Geometry: final body of the model. Coordinates: model frame, mm. Face numbers are marked on the shaded views. A direction names the side the tool comes from. Coordinates: 2 decimals unless noted, no trailing zeros. Loops run counter-clockwise (first coordinate to the right, second up) from the corner with the lowest first, then second, coordinate; pieces in that order, holes last. Notation, with made-up numbers: (58, 47) -> (88, 47) arc R27 cw to (88, 79) -> close; hole circle Ø2 at (72, -26). An arc over 180 degrees is marked (long way). One line per item, written item: value. Start each with the question number.
Item 1: Set-up query: the marked faces 1, 2, 3, 4 and 5. Return all of +Z, -Z, +X, -X, +Y, -Y with unobstructed straight access to the full face (end or side cutting, diameter ignored); none if empty.
Item 2: Section query C-C on x = 2.3. Return loops of the section in (y, z).
Item 3: Section query A-A on x = 3. Return loops of the section in (y, z), then the cut area to 3 significant figures.
Item 4: Section query D-D on x = -0.9. Return loops of the section in (y, z), then the cut area to 3 significant figures.
Item 5: Section query B-B on z = 1.55. Return loops of the section in (x, y).
Item 6: Ray query, probe 1 along Y at (x, z) = (2.1, 2.7); probe 2 along X at (y, z) = (-1.8, 0.2); probe 3 along Z at (x, y) = (1.35, 2.15). Return the intervals inside material, ascending. Write a range as from..to.
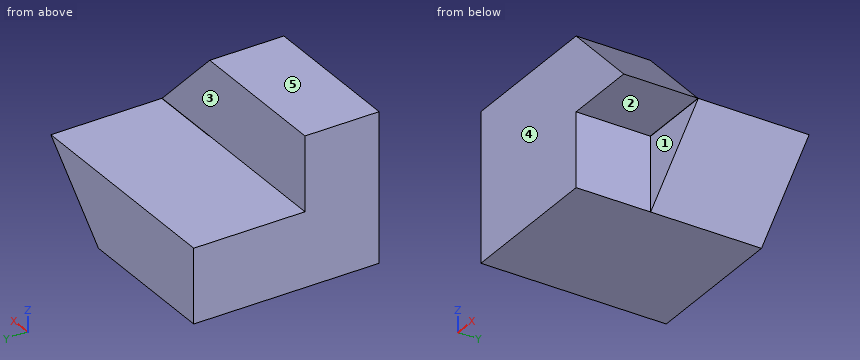
from build123d import *

# Parameters (mm, degrees)
SKETCH1_W           = 4
SKETCH1_H           = 5
BOSS_EXTRUDE1_DEPTH = 2
SKETCH2_W           = 4
SKETCH2_H           = 2
BOSS_EXTRUDE2_DEPTH = 2
BOSS_EXTRUDE3_DEPTH = 2
BOSS_EXTRUDE5_DEPTH = 2.99


with BuildPart() as part:
    # Sketch1 → Boss-Extrude1 (new body)
    with BuildSketch(Plane.XY):
        Rectangle(SKETCH1_W, SKETCH1_H)
    extrude(amount=BOSS_EXTRUDE1_DEPTH)

    # Sketch2 → Boss-Extrude2 (add)
    with BuildSketch(Plane.XY.offset(2)):
        with Locations((0, -1.5)):
            Rectangle(SKETCH2_W, SKETCH2_H)
    extrude(amount=BOSS_EXTRUDE2_DEPTH)

    # Sketch3 → Boss-Extrude3 (add)
    with BuildSketch(Plane(origin=(0, -0.5, 0), x_dir=(1, 0, 0), z_dir=(0, 1, 0))):
        Polygon((2, -4), (4, -2), (2, -2), align=None)
    extrude(amount=-BOSS_EXTRUDE3_DEPTH)

    # Sketch5 → Boss-Extrude5 (add)
    with BuildSketch(Plane(origin=(0, 2.5, 0), x_dir=(1, 0, 0), z_dir=(0, 1, 0))):
        Polygon((2, 0), (4, -2), (2, -2), align=None)
    extrude(amount=-BOSS_EXTRUDE5_DEPTH)


solid = part.part
Reply:
1. face 1: +Z, -Z, +X, -Y
1. face 2: -Z, +X, -Y
1. face 3: +Z, +X, -X, +Y
1. face 4: +Z, -Z, +X, -X, -Y
1. face 5: +Z, +X, -X, +Y, -Y
2. outline: (-2.5, 2) -> (-0.5, 2) -> (-0.5, 3.7) -> (-2.5, 3.7) -> close; (-0.49, 0.3) -> (2.5, 0.3) -> (2.5, 2) -> (-0.49, 2) -> close
3. outline: (-2.5, 2) -> (-0.5, 2) -> (-0.5, 3) -> (-2.5, 3) -> close; (-0.49, 1) -> (2.5, 1) -> (2.5, 2) -> (-0.49, 2) -> close
3. area: 4.99 mm²
4. outline: (-2.5, 0) -> (2.5, 0) -> (2.5, 2) -> (-0.5, 2) -> (-0.5, 4) -> (-2.5, 4) -> close
4. area: 14.0 mm²
5. outline: (-2, -2.5) -> (2, -2.5) -> (2, -0.49) -> (3.55, -0.49) -> (3.55, 2.5) -> (-2, 2.5) -> close
6. probe 1: y = -2.5..-0.5
6. probe 2: x = -2..2
6. probe 3: z = 0..2
